Design review of the part built by this model. Coordinates are the model's own, in mm. A direction names the side the tool comes from. Round coordinates to 2 decimals unless told otherwise and drop trailing zeros. Loops run counter-clockwise (first coordinate to the right, second up) from the corner with the lowest first, then second, coordinate; pieces in that order, holes last. Notation, with made-up numbers: (-38, 9) - (-6, 9) arc R12 cw to (-6, 18) - close; hole circle Ø2 at (18.25, 39.5). An arc over 180 degrees is marked (long way). Return JSON: item names as keys, results as strings. Group by question number.
from build123d import *

# Parameters (mm, degrees)
F0_W     = 42.4149371684
F0_H     = 38.9721691608
F1_DEPTH = 25.4
F5_DEPTH = 25


# Not quite as in the source:
# - the program builds the solid bodies; features that only make, move or delete a surface that nothing else refers to are left out


with BuildPart() as f1:
    # F0 (on Front) → F1 (new body)
    with BuildSketch(Plane.XZ):
        with Locations((21.2074685842, 19.4860845804)):
            Rectangle(F0_W, F0_H)
    extrude(amount=F1_DEPTH)

    # F4 (on face) → F5 (cut)
    with BuildSketch(Plane.XZ.offset(25.4)):
        with BuildLine():
            ThreePointArc((19.4994620307, 22.614925386), (18.3126908163, 5.6894142875), (33.200540329, 13.8277979568))
            ThreePointArc((33.200540329, 13.8277979568), (33.1944083659, 14.1720857887), (33.176020255, 14.5159369041))
            ThreePointArc((33.176020255, 14.5159369041), (23.8873414039, 14.4275027139), (19.4994620307, 22.614925386))
        make_face()
    extrude(amount=-F5_DEPTH, mode=Mode.SUBTRACT)


solid = f1.part
Q1. For line 1 (Z direction, x = 15.5, y = -6.25); line 2 (Z direction, x = 22.5, y = -1.75); line 3 (X direction, y = -15.5, z = 11.5), list the stretches that pass through material, from the lowest coordinate up.
Q2. Tool access review of faces 5 (the flat face through (21, -0.4, 11)), 6 (the flat face through (21, -25.4, 20)): name each direction out of +Z, -Z, +X, -X, +Y, -Y from which nothing blocks a thin tool from reaching the whole face with its end or side.
Q3. Add section A-A, the plane z = 7.5. State the section outline as (x, y) points.
Q4. Add section C-C, the plane x = 17.5. State the section outline as (y, z) points.
Q5. Add section B-B, the plane y = -6.25. State the section outline as (x, z) points, plus the area to 3 significant figures.
Q6. Draft analysis for pull direction Z (two halves, no side actions). For faces 1 (the flat face through (21, -13, 38.972)), 2 (the cylindrical face through (24.005, -13.075, 14.359)), 3 (the flat face through (21, 0, 20)), 4 (the flat face through (21, -13, 0)), state which applies: pulls with the +Z half, pulls with the -Z half, needs draft (parallel to the pull), parting line crosses it, or undercut.
Evaluation:
{
 "1": {"line 1": "0 to 8.45, 19.21 to 38.97", "line 2": "0 to 4.21, 15.44 to 38.97", "line 3": "0 to 14.15, 32.92 to 42.41"},
 "2": {"face 5": "-Y", "face 6": "+Z, -Z, +X, -X, -Y"},
 "3": {"outline": "(0, -25.4) - (16.22, -25.4) - (16.22, -0.4) - (30.84, -0.4) - (30.84, -25.4) - (42.41, -25.4) - (42.41, 0) - (0, 0) - close"},
 "4": {"outline": "(-25.4, 0) - (0, 0) - (0, 38.97) - (-25.4, 38.97) - (-25.4, 21.38) - (-0.4, 21.38) - (-0.4, 6.27) - (-25.4, 6.27) - close"},
 "5": {"outline": "(0, 0) - (42.41, 0) - (42.41, 38.97) - (0, 38.97) - close; hole (19.5, 22.61) arc R9.67 ccw (long way) to (33.18, 14.52) arc R8.97 cw to start", "area": "1,460 mm²"},
 "6": {"face 1": "pulls with the +Z half", "face 2": "undercut", "face 3": "needs draft", "face 4": "pulls with the -Z half"}
}
